from build123d import *

# Parameters (mm, degrees)
SKETCH_1_R          = 1.65
SKETCH_1_R_2        = 1.6
SKETCH_1_R_3        = 12
EXTRUDE_2_DEPTH     = 7
CUT_EXTRUDE_1_DEPTH = 4
CHAMFER_1_SIZE      = 1.5


with BuildPart() as part:
    # Эскиз1 → Бобышка-Вытянуть2 (new body)
    with BuildSketch(Plane(origin=(0, 0, 0), x_dir=(1, 0, 0), z_dir=(0, 1, 0))):
        with BuildLine():
            ThreePointArc((-18.152308777, -11.756549774), (-19.411562194, -13.145772627), (-20, -14.926053575))
            Line((-20, -14.926053575), (-20, -15.926053575))
            ThreePointArc((-20, -15.926053575), (-18.535533906, -19.461587481), (-15, -20.926053575))
            Line((-15, -20.926053575), (15, -20.926053575))
            ThreePointArc((15, -20.926053575), (18.535533906, -19.461587481), (20, -15.926053575))
            Line((20, -15.926053575), (20, -14.926053575))
            ThreePointArc((20, -14.926053575), (19.411562194, -13.145772627), (18.152308777, -11.756549774))
            ThreePointArc((18.152308777, -11.756549774), (16.300607831, -9.168856683), (16.385075524, -5.988005046))
            ThreePointArc((16.385075524, -5.988005046), (17.444900664, 0.048427023), (16.351577861, 6.078881955))
            ThreePointArc((16.351577861, 6.078881955), (16.257522585, 9.285823976), (18.131827713, 11.889725627))
            ThreePointArc((18.131827713, 11.889725627), (19.405196174, 13.282780162), (20, 15.073946425))
            Line((20, 15.073946425), (20, 16.073946425))
            ThreePointArc((20, 16.073946425), (18.535533906, 19.609480331), (15, 21.073946425))
            Line((15, 21.073946425), (-15, 21.073946425))
            ThreePointArc((-15, 21.073946425), (-18.535533906, 19.609480331), (-20, 16.073946425))
            Line((-20, 16.073946425), (-20, 15.073946425))
            ThreePointArc((-20, 15.073946425), (-19.405196174, 13.282780162), (-18.131827713, 11.889725627))
            ThreePointArc((-18.131827713, 11.889725627), (-16.257522585, 9.285823976), (-16.351577861, 6.078881955))
            ThreePointArc((-16.351577861, 6.078881955), (-17.444900664, 0.048427023), (-16.385075524, -5.988005046))
            ThreePointArc((-16.385075524, -5.988005046), (-16.300607831, -9.168856683), (-18.152308777, -11.756549774))
        make_face()
        with Locations((-15.5, -15.426053575)):
            Circle(SKETCH_1_R, mode=Mode.SUBTRACT)
        with Locations((-8, -17.426053575)):
            Circle(SKETCH_1_R_2, mode=Mode.SUBTRACT)
        with Locations((15.5, -15.426053575)):
            Circle(SKETCH_1_R, mode=Mode.SUBTRACT)
        Circle(SKETCH_1_R_3, mode=Mode.SUBTRACT)
        with Locations((-15.5, 15.573946425)):
            Circle(SKETCH_1_R, mode=Mode.SUBTRACT)
        with Locations((-8, 17.573946425)):
            Circle(SKETCH_1_R_2, mode=Mode.SUBTRACT)
        with Locations((15.5, 15.573946425)):
            Circle(SKETCH_1_R, mode=Mode.SUBTRACT)
    extrude(amount=EXTRUDE_2_DEPTH)

    # Эскиз2 → Вырез-Вытянуть1 (cut)
    with BuildSketch(Plane(origin=(0, 7, 0), x_dir=(1, 0, 0), z_dir=(0, 1, 0))):
        Polygon((-11.348631561, 17.573946425), (-9.674315781, 14.673946425), (-6.325684219, 14.673946425), (-4.651368439, 17.573946425), (-6.325684219, 20.473946425), (-9.674315781, 20.473946425), align=None)
        Polygon((-4.651368439, -17.426053575), (-6.325684219, -14.526053575), (-9.674315781, -14.526053575), (-11.348631561, -17.426053575), (-9.674315781, -20.326053575), (-6.325684219, -20.326053575), align=None)
    extrude(amount=-CUT_EXTRUDE_1_DEPTH, mode=Mode.SUBTRACT)

    # Фаска1
    chamfer_1_edges = [part.edges().sort_by_distance(p)[0] for p in [
        (-17.15, 0, 15.426053575),
        (13.85, 0, 15.426053575),
        (13.85, 0, -15.573946425),
        (-17.15, 0, -15.573946425),
    ]]
    chamfer(chamfer_1_edges, length=CHAMFER_1_SIZE)


solid = part.part
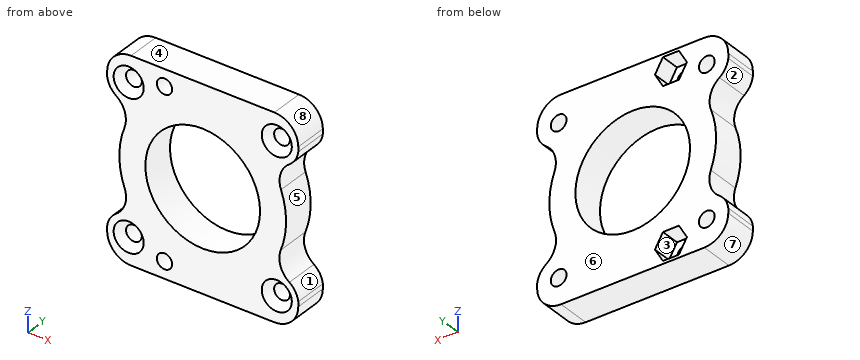
Can you work these out from the model? Positions are in its coordinate system, mm. Face numbers are marked on the shaded views. A direction names the side the tool comes from. Coordinates: 2 decimals unless noted, no trailing zeros. Write each loop counter-clockwise with the first axis right and the second up, starting at its lowest first coordinate (ties: lowest second). Pieces come first, ordered by that corner, then holes. Notation, with made-up numbers: (79.5, 86.5) - (137.5, 86.5) arc R5 ccw to (137.5, 93.5) - close; hole circle Ø2 at (6, 52). An arc over 180 degrees is marked (long way). Return JSON: item names as keys, results as strings. Group by question number.
Item 1: If we section it at C-C (x = -8.5): Write out the boundary of the cut face in (y, z), then the cut area to 3 significant figures.
Item 2: If we section it at B-B (z = 0): Write out the boundary of the cut face in (x, y).
Item 3: Which directions (+Z, -Z, +X, -X, +Y, -Y) give clear straight access to the entire face, cutting with the end or side of a thin tool? Please do the marked faces 1, 2, 3 and 4.
Item 4: If we section it at A-A (x = 0): Write out the boundary of the cut face in (y, z), then the cut area to 3 significant figures.
Item 5: I'm going to push flat-ended pins straight in: pin 1 Ø4 at (x, z) = (15.5, 15.43) entering from -Y; pin 2 Ø1.5 at (y, z) = (5.5, -9.5) entering from +X. Where does each tip first touch, or does it pass through?
Item 6: If we section it at D-D (x = -15.5): Write out the boundary of the cut face in (y, z), then the cut area to 3 significant figures.
Item 7: Please list where these lines run through material, in increasing order: probe 1 along Z at (x, y) = (0, 3.75); probe 2 along X at (y, z) = (5.25, 0); probe 3 along Z at (x, y) = (-15.5, 4.25).
Item 8: We'd pull the mould along Z, two halves only. Please class the marked faces 5, 6, 7 and 8: pulls with the +Z half, pulls with the -Z half, needs draft (parallel to the pull), parting line crosses it, or undercut.
Return value:
{
 "1": {"outline": "(0, -21.07) - (7, -21.07) - (7, -20.47) - (3, -20.47) - (3, -19.09) - (0, -19.09) - close; (0, -16.05) - (3, -16.05) - (3, -14.67) - (7, -14.67) - (7, -8.47) - (0, -8.47) - close; (0, 8.47) - (7, 8.47) - (7, 14.53) - (3, 14.53) - (3, 15.91) - (0, 15.91) - close; (0, 18.95) - (3, 18.95) - (3, 20.33) - (7, 20.33) - (7, 20.93) - (0, 20.93) - close", "area": "111 mm^2"},
 "2": {"outline": "(-17.44, 0) - (-12, 0) - (-12, 7) - (-17.44, 7) - close; (12, 0) - (17.44, 0) - (17.44, 7) - (12, 7) - close"},
 "3": {"face 1": "+X, +Y, -Y", "face 2": "-X, +Y, -Y", "face 3": "+Y", "face 4": "+Z, +X, -X, +Y, -Y"},
 "4": {"outline": "(0, -21.07) - (7, -21.07) - (7, -12) - (0, -12) - close; (0, 12) - (7, 12) - (7, 20.93) - (0, 20.93) - close", "area": "126 mm^2"},
 "5": {"pin 1": "stops at y = 1.15", "pin 2": "stops at x = 16.67"},
 "6": {"outline": "(0, -21.05) - (7, -21.05) - (7, -17.22) - (1.5, -17.22) - (0, -18.72) - close; (0, -12.42) - (1.5, -13.92) - (7, -13.92) - (7, 13.78) - (1.5, 13.78) - (0, 12.28) - close; (0, 18.58) - (1.5, 17.08) - (7, 17.08) - (7, 20.9) - (0, 20.9) - close", "area": "243 mm^2"},
 "7": {"probe 1": "z = -21.07 to -12, 12 to 20.93", "probe 2": "x = -17.44 to -12, 12 to 17.44", "probe 3": "z = -21.05 to -17.22, -13.92 to 13.78, 17.08 to 20.9"},
 "8": {"face 5": "undercut", "face 6": "needs draft", "face 7": "pulls with the -Z half", "face 8": "pulls with the +Z half"}
}
